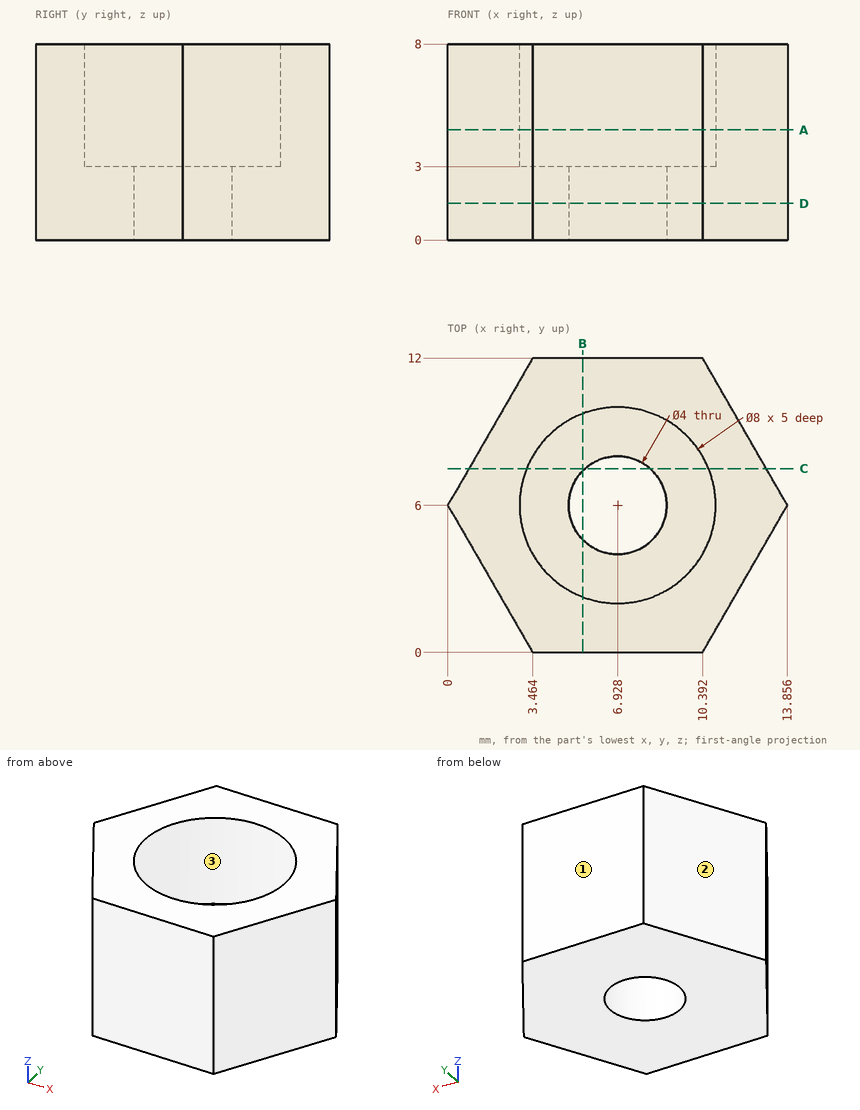
The drawing under review shows one solid part. Ordinate dimensions are in mm from its lowest x, y, z. Coordinates: 2 decimals unless noted, no trailing zeros. Write each loop counter-clockwise with the first axis right and the second up, starting at its lowest first coordinate (ties: lowest second). Pieces come first, ordered by that corner, then holes.
1) Add section A-A (z = 4.5). Write out the cut boundary in (x, y).
2) Mouldability with a two-part tool opening along X and no side actions: class the marked faces 1, 2 and 3 as +X half, -X half, draft (parallel to the pull), parting line (faces both ways), or undercut.
3) Add section C-C (y = 7.5). Write out the cut boundary in (x, z) (1 decimal).
4) Add section D-D (z = 1.5). Write out the cut boundary in (x, y).
5) Add section B-B (x = 5.5). Write out the cut boundary in (y, z).
6) Insertion check: pin 1 (1.5 mm diameter, centred on y = 9.5, z = 5.5, fed in from -X); pin 2 (6.5 mm diameter, centred on x = 6.5, y = 6, fed in from +Z); pin 3 (2.5 mm diameter, centred on x = 6.93, y = 6, fed in from +Z). Each pin has a flat end and moves straight along its axis. Give the tip position at first contact, or say it passes through.
7) To check wall thickness, follow L1, parallel to Z at x = 8.5, y = 8.25; L2, parallel to Y at x = 5.25, z = 7; L3, parallel to X at y = 6.75, z = 4.5 (1 decimal). State the ranges of each line that lie inside material, in increasing order.
Check result:
1. outline: (0, 6) - (3.46, 0) - (10.39, 0) - (13.86, 6) - (10.39, 12) - (3.46, 12) - close; hole circle Ø8 at (6.93, 6)
2. face 1: draft
2. face 2: -X half
2. face 3: undercut
3. outline: (0.9, 0) - (5.6, 0) - (5.6, 3) - (3.2, 3) - (3.2, 8) - (0.9, 8) - close; (8.3, 0) - (13, 0) - (13, 8) - (10.6, 8) - (10.6, 3) - (8.3, 3) - close
4. outline: (0, 6) - (3.46, 0) - (10.39, 0) - (13.86, 6) - (10.39, 12) - (3.46, 12) - close; hole circle Ø4 at (6.93, 6)
5. outline: (0, 0) - (4.6, 0) - (4.6, 3) - (2.26, 3) - (2.26, 8) - (0, 8) - close; (7.4, 0) - (12, 0) - (12, 8) - (9.74, 8) - (9.74, 3) - (7.4, 3) - close
6. pin 1: stops at x = 1.59
6. pin 2: stops at z = 3
6. pin 3: passes through
7. L1: z = 0 to 3
7. L2: y = 0 to 2.37, 9.63 to 12
7. L3: x = 0.4 to 3, 10.9 to 13.4
